For this review, take the finished solid that the model builds, in its own axes (mm). Face numbers are marked on the shaded views. A direction names the side the tool comes from. Give positions to 0.01 mm unless a question says otherwise; leave off trailing zeros. Write each loop counter-clockwise with the first axis right and the second up, starting at its lowest first coordinate (ties: lowest second). Pieces come first, ordered by that corner, then holes. Notation, with made-up numbers: (53.5, 26) -> (93.5, 26) arc R12 ccw to (93.5, 34) -> close; hole circle Ø1 at (-38, 23.5). An arc over 180 degrees is marked (long way). Return JSON: item names as keys, results as strings.
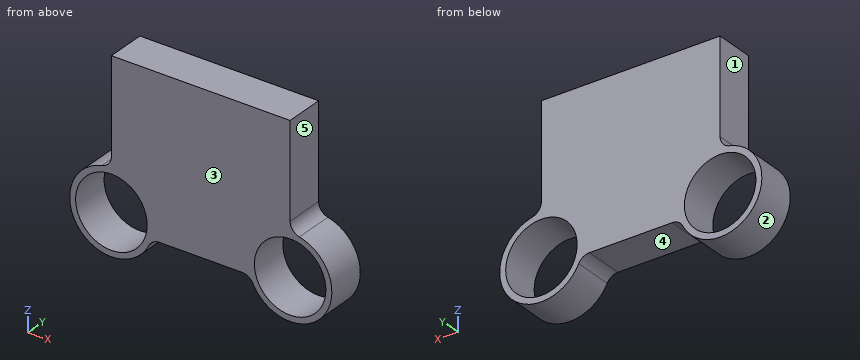
from build123d import *

# Parameters (mm, degrees)
SKETCH1_R           = 30
BOSS_EXTRUDE1_DEPTH = 33
FILLET1_R           = 10


with BuildPart() as part:
    # Sketch1 → Boss-Extrude1 (new body)
    with BuildSketch(Plane(origin=(0, 0, 0), x_dir=(1, 0, 0), z_dir=(0, 1, 0))):
        with BuildLine():
            Line((75, 0), (-75, 0))
            Line((-75, 0), (-75, 88))
            ThreePointArc((-75, 88), (-103.062430401, 143.916500663), (-41.458980338, 133))
            Line((-41.458980338, 133), (41.458980338, 133))
            ThreePointArc((41.458980338, 133), (103.062430401, 143.916500663), (75, 88))
            Line((75, 88), (75, 0))
        make_face()
        with Locations((-75, 123)):
            Circle(SKETCH1_R, mode=Mode.SUBTRACT)
        with Locations((75, 123)):
            Circle(SKETCH1_R, mode=Mode.SUBTRACT)
    extrude(amount=BOSS_EXTRUDE1_DEPTH)

    # Fillet1
    fillet1_edges = [part.edges().sort_by_distance(p)[0] for p in [
        (-75, 16.5, -88),
        (-41.458980338, 16.5, -133),
        (41.458980338, 16.5, -133),
        (75, 16.5, -88),
    ]]
    fillet(fillet1_edges, radius=FILLET1_R)


solid = part.part
1. Add section C-C, the plane y = 29. State the section outline as (x, z) points, plus the area to 3 significant figures.
Results found:
{"outline": "(-82.78, -88.88) arc R35 ccw (long way) to (-43.65, -138.56) arc R10 cw to (-34.69, -133) -> (34.69, -133) arc R10 cw to (43.65, -138.56) arc R35 ccw (long way) to (82.78, -88.88) arc R10 cw to (75, -79.13) -> (75, 0) -> (-75, 0) -> (-75, -79.13) arc R10 cw to start; hole circle Ø60 at (-75, -123); hole circle Ø60 at (75, -123)", "area": "19,400 mm²"}
2. For pin 1 (10 mm diameter, centred on x = 4.5, y = 19, fed in from -Z); pin 2 (8 mm diameter, centred on y = 16.5, z = -99.5, fed in from +X); pin 3 (12 mm diameter, centred on y = 6, z = -42.5, fed in from +X), all flat-tipped, find the tip position at first contact; note any pin that passes through.
Results found:
{"pin 1": "stops at z = -133", "pin 2": "stops at x = 104.06", "pin 3": "stops at x = 75"}
3. For the marked faces 1 and 2, list the 3-axis set-ups (+Z, -Z, +X, -X, +Y, -Y) from which the entire face can be reached by the end or side of a thin tool; tool diameter is ignored.
Results found:
{"face 1": "+Z, -X, +Y, -Y", "face 2": "+Y, -Y"}
4. The part is to be moulded in two halves that separate along X. For the marked faces 3, 4 and 5, say which applies: +X half, -X half, draft (parallel to the pull), parting line (faces both ways), or undercut.
Results found:
{"face 3": "draft", "face 4": "undercut", "face 5": "+X half"}
5. Add section B-B, the plane x = -48. State the section outline as (y, z) points.
Results found:
{"outline": "(0, -145.27) -> (33, -145.27) -> (33, -136.08) -> (0, -136.08) -> close; (0, -109.92) -> (33, -109.92) -> (33, 0) -> (0, 0) -> close"}
6. Add section D-D, the plane z = -142. State the section outline as (x, y) points, plus the area to 3 significant figures.
Results found:
{"outline": "(-104.39, 0) -> (-98.22, 0) -> (-98.22, 33) -> (-104.39, 33) -> close; (-51.78, 0) -> (-45.61, 0) -> (-45.61, 33) -> (-51.78, 33) -> close; (45.61, 0) -> (51.78, 0) -> (51.78, 33) -> (45.61, 33) -> close; (98.22, 0) -> (104.39, 0) -> (104.39, 33) -> (98.22, 33) -> close", "area": "815 mm²"}
7. Add section A-A, the plane z = -123. State the section outline as (x, y) points, plus the area to 3 significant figures.
Results found:
{"outline": "(-110, 0) -> (-105, 0) -> (-105, 33) -> (-110, 33) -> close; (-45, 0) -> (45, 0) -> (45, 33) -> (-45, 33) -> close; (105, 0) -> (110, 0) -> (110, 33) -> (105, 33) -> close", "area": "3,300 mm²"}
8. To check wall thickness, follow probe 1 along X at (y, z) = (11, -123); probe 2 along X at (y, z) = (27, -120); probe 3 along X at (y, z) = (19, -77). State the ranges of each line that lie inside material, in increasing order.
Results found:
{"probe 1": "x = -110 to -105, -45 to 45, 105 to 110", "probe 2": "x = -109.87 to -104.85, -45.15 to 45.15, 104.85 to 109.87", "probe 3": "x = -75 to 75"}
